Job drawing, mm, ordinate dimensions from the low corner. One solid piece. A direction names the side the tool comes from. Round coordinates to 2 decimals unless told otherwise and drop trailing zeros. Loops run counter-clockwise (first coordinate to the right, second up) from the corner with the lowest first, then second, coordinate; pieces in that order, holes last. Notation, with made-up numbers: M -15,3.25 L -1,3.25 A32 cw -1,38.25 Z; hole C 69,12 d1. An arc over 180 degrees is marked long. One line per item, written item: value.
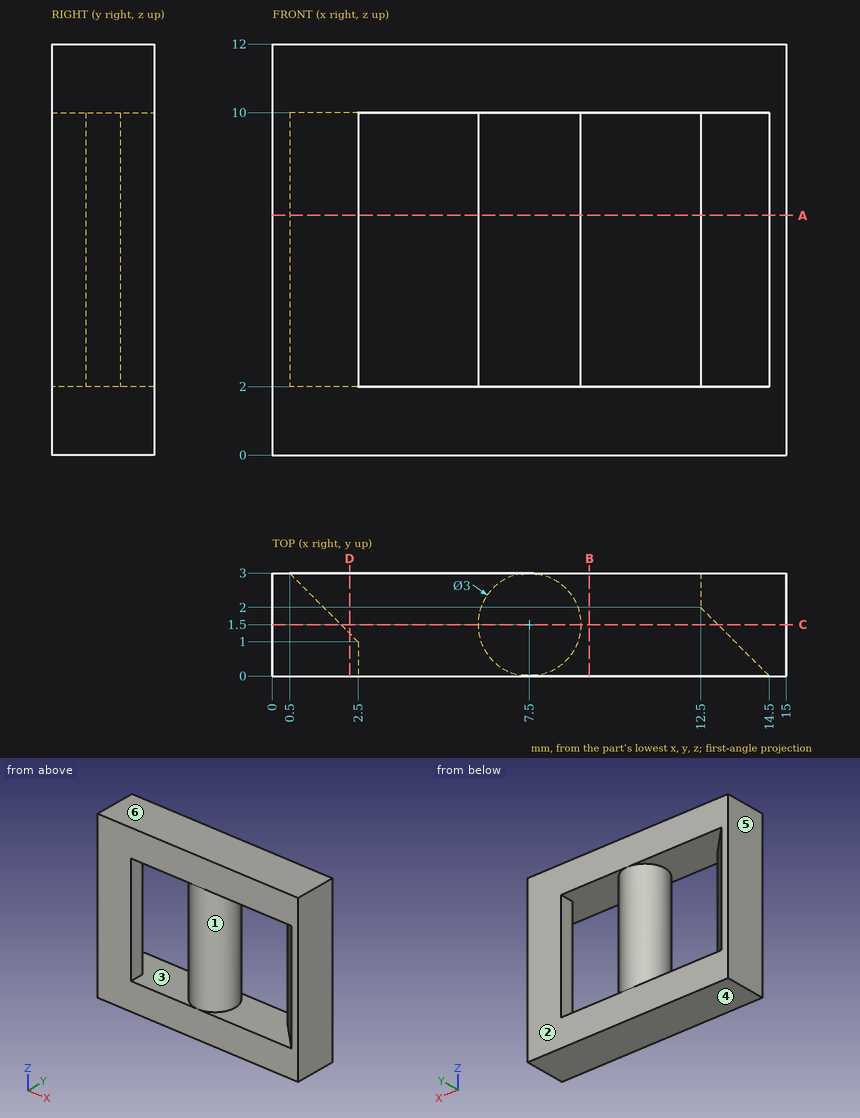
Item 1: Slice it at D-D, the plane x = 2.25. Give the cut face in (y, z), and give its area (3 significant figures).
Check values:
outline: M 0,0 L 3,0 L 3,2 L 1.25,2 L 1.25,10 L 3,10 L 3,12 L 0,12 Z
area: 22.0 mm2
Item 2: Slice it at A-A, the plane z = 7. Give the cut face in (x, y), and give its area (3 significant figures).
Check values:
outline: M 0,0 L 2.5,0 L 2.5,1 L 0.5,3 L 0,3 Z; C 7.5,1.5 d3; M 12.5,2 L 14.5,0 L 15,0 L 15,3 L 12.5,3 Z
area: 18.1 mm2
Item 3: Slice it at C-C, the plane y = 1.5. Give the cut face in (x, z), and give its area (3 significant figures).
Check values:
outline: M 0,0 L 15,0 L 15,12 L 0,12 Z; hole M 2,2 L 6,2 L 6,10 L 2,10 Z; hole M 9,2 L 13,2 L 13,10 L 9,10 Z
area: 116 mm2
Item 4: Pull direction Z, two halves, no side cores. Call the marked faces 3, 4, 5 and 6: pulls with the +Z half, pulls with the -Z half, needs draft (parallel to the pull), parting line crosses it, or undercut.
Check values:
face 3: undercut
face 4: pulls with the -Z half
face 5: needs draft
face 6: pulls with the +Z half
Item 5: Wall check: line 1 along Z through (x, y) = (12.5, 1.7); line 2 along X through (y, z) = (0.75, 7); line 3 along X through (y, z) = (2.4, 6). Give the ranges that are in metal, low to high.
Check values:
line 1: z = 0 to 2, 10 to 12
line 2: x = 0 to 2.5, 6.2 to 8.8, 13.75 to 15
line 3: x = 0 to 1.1, 6.3 to 8.7, 12.5 to 15
Item 6: Which spindle directions (+Z, -Z, +X, -X, +Y, -Y) get a long thin tool onto all of the face, cutting with end or side? Do the marked faces 1 and 2. Say none if no direction does.
Check values:
face 1: none
face 2: +Z, -Z, +X, -X, +Y
Item 7: Drop a flat-ended pin along its axis: P1, Ø1.5, axis at x = 6, z = 9, coming from the +Y side. Give the stop position or say it passes through.
Check values:
P1: stops at y = 2.8
Item 8: Slice it at B-B, the plane x = 9.25. Give the cut face in (y, z).
Check values:
outline: M 0,0 L 3,0 L 3,2 L 0,2 Z; M 0,10 L 3,10 L 3,12 L 0,12 Z
